For this review, take the finished solid that the model builds, in its own axes (mm). A direction names the side the tool comes from. Coordinates: 2 decimals unless noted, no trailing zeros. Loops run counter-clockwise (first coordinate to the right, second up) from the corner with the lowest first, then second, coordinate; pieces in that order, holes last. Notation, with made-up numbers: (-31, -0.75) -> (-14, -0.75) arc R34 ccw to (-14, 38.25) -> close; hole circle Ø2 at (46, -29). An arc over 180 degrees is marked (long way). Use a Markdown table: item, result.
from build123d import *

# Parameters (mm, degrees)
MODEL_R                 = 1.5
SALIENTE_EXTRUIR1_DEPTH = 3


with BuildPart() as part:
    # Model → Saliente-Extruir1 (new body)
    with BuildSketch(Plane.XY):
        with BuildLine():
            Line((132.104752837, 242.341546665), (132.104752837, 236.341546665))
            Line((132.104752837, 236.341546665), (133.604752837, 236.341546665))
            ThreePointArc((133.604752837, 236.341546665), (134.665413008, 235.902206837), (135.104752837, 234.841546665))
            Line((135.104752837, 234.841546665), (135.104752837, 233.341546665))
            Line((135.104752837, 233.341546665), (143.604752837, 233.341546665))
            Line((143.604752837, 233.341546665), (143.604752837, 234.841546665))
            ThreePointArc((143.604752837, 234.841546665), (144.044092665, 235.902206837), (145.104752837, 236.341546665))
            Line((145.104752837, 236.341546665), (146.604752837, 236.341546665))
            Line((146.604752837, 236.341546665), (146.604752837, 242.341546665))
            Line((146.604752837, 242.341546665), (145.104752837, 242.341546665))
            ThreePointArc((145.104752837, 242.341546665), (144.044092665, 242.780886493), (143.604752837, 243.841546665))
            Line((143.604752837, 243.841546665), (143.604752837, 245.341546665))
            Line((143.604752837, 245.341546665), (135.104752837, 245.341546665))
            Line((135.104752837, 245.341546665), (135.104752837, 243.841546665))
            ThreePointArc((135.104752837, 243.841546665), (134.665413008, 242.780886493), (133.604752837, 242.341546665))
            Line((133.604752837, 242.341546665), (132.104752837, 242.341546665))
        make_face()
        with Locations((139.354752837, 239.341546665)):
            Circle(MODEL_R, mode=Mode.SUBTRACT)
    extrude(amount=SALIENTE_EXTRUIR1_DEPTH)


solid = part.part
(1) For pin 1 Ø1.2 at (x, z) = (146, 1) entering from -Y; pin 2 Ø1 at (x, z) = (134, 0.5) entering from +Y; pin 3 Ø1.2 at (y, z) = (244.5, 2) entering from +X; pin 4 Ø2.5 at (x, y) = (139.35, 239.34) entering from +Z, all flat-tipped, find the tip position at first contact; note any pin that passes through.
Found:
| item | result |
|---|---|
| pin 1 | stops at y = 236.34 |
| pin 2 | stops at y = 242.64 |
| pin 3 | stops at x = 143.6 |
| pin 4 | passes through |
(2) Take a section at D-D on x = 145.5. Write out the cut boundary in (y, z), plus the area to 3 significant figures.
Found:
| item | result |
|---|---|
| outline | (236.34, 0) -> (242.34, 0) -> (242.34, 3) -> (236.34, 3) -> close |
| area | 18.0 mm^2 |
(3) Take a section at C-C on z = 1.05. Write out the cut boundary in (x, y).
Found:
| item | result |
|---|---|
| outline | (132.1, 236.34) -> (133.6, 236.34) arc R1.5 cw to (135.1, 234.84) -> (135.1, 233.34) -> (143.6, 233.34) -> (143.6, 234.84) arc R1.5 cw to (145.1, 236.34) -> (146.6, 236.34) -> (146.6, 242.34) -> (145.1, 242.34) arc R1.5 cw to (143.6, 243.84) -> (143.6, 245.34) -> (135.1, 245.34) -> (135.1, 243.84) arc R1.5 cw to (133.6, 242.34) -> (132.1, 242.34) -> close; hole circle Ø3 at (139.35, 239.34) |
(4) For faces 4 (the face through (135.105, 245, 1)), 5 (the face through (143.605, 234, 1)), 6 (the face through (133, 236.342, 1)), 7 (the face through (143.605, 245, 1)), list the 3-axis set-ups (+Z, -Z, +X, -X, +Y, -Y) from which the entire face can be reached by the end or side of a thin tool; tool diameter is ignored.
Found:
| item | result |
|---|---|
| face 4 | +Z, -Z, -X, +Y |
| face 5 | +Z, -Z, +X, -Y |
| face 6 | +Z, -Z, -X, -Y |
| face 7 | +Z, -Z, +X, +Y |
(5) Take a section at B-B on y = 238.5. Write out the cut boundary in (x, z).
Found:
| item | result |
|---|---|
| outline | (132.1, 0) -> (138.11, 0) -> (138.11, 3) -> (132.1, 3) -> close; (140.6, 0) -> (146.6, 0) -> (146.6, 3) -> (140.6, 3) -> close |
(6) Mouldability with a two-part tool opening along X and no side actions: class faces 1 (the face through (144.03, 235.89, 1.48)), 2 (the face through (139.03, 237.877, 1.479)), 3 (the face through (133, 242.342, 1)) as pulls with the +X half, pulls with the -X half, needs draft (parallel to the pull), parting line crosses it, or undercut.
Found:
| item | result |
|---|---|
| face 1 | pulls with the +X half |
| face 2 | undercut |
| face 3 | needs draft |
(7) For line 1 along Y through (x, z) = (145.5, 2.2); line 2 along X through (y, z) = (239, 2.8); line 3 along X through (y, z) = (240, 0.45), list the stretches that pass through material, from the lowest coordinate up.
Found:
| item | result |
|---|---|
| line 1 | y = 236.34 to 242.34 |
| line 2 | x = 132.1 to 137.89, 140.82 to 146.6 |
| line 3 | x = 132.1 to 138.01, 140.7 to 146.6 |
(8) Take a section at A-A on x = 138.25. Write out the cut boundary in (y, z).
Found:
| item | result |
|---|---|
| outline | (233.34, 0) -> (238.33, 0) -> (238.33, 3) -> (233.34, 3) -> close; (240.36, 0) -> (245.34, 0) -> (245.34, 3) -> (240.36, 3) -> close |
